Check sheet for the modelled part. Datum: model origin and axes. Units: mm. A direction names the side the tool comes from. Round coordinates to 2 decimals unless told otherwise and drop trailing zeros. Order: outer loops, then holes, each group sorted by start corner. A loop starts at its lowest first (then second) coordinate and runs counter-clockwise, first axis right, second up. Notation, with made-up numbers: (89.5, -2) -> (145.5, -2) arc R21 cw to (145.5, 8) -> close; hole circle Ø11 at (-5, 84). An arc over 180 degrees is marked (long way). Answer in a Markdown table with one row per item. Add a question column.
1. Draft check along Z on faces 4 (the flat face through (-1, 6, -22.23)), 5 (the flat face through (9.336, -0.986, 2.65)), 6 (the flat face through (38.655, 6, 0)), 7 (the cylindrical face through (26.151, 8.338, -18.804)). Enter one of: +Z half, -Z half, draft (parallel to the pull), parting line (faces both ways), or undercut.
2. Material ranges on L1, parallel to X at y = 9, z = -11 (3 decimals); L2, parallel to X at y = 6.25, z = -15.5 (3 decimals); L3, parallel to X at y = 13.75, z = -4.5 (3 decimals), recorded low to high. Write a range as from..to.
3. Sectioned sample at C-C, the plane z = 17. Record the boundary of the cut face in (x, y) (3 decimals), then the cut area to 3 significant figures.
4. Sectioned sample at D-D, the plane x = -14.5. Record the boundary of the cut face in (y, z).
5. Depth check by flat-ended pin: P1, Ø10, axis at x = 23.5, z = -15, coming from the -Y side; P2, Ø0.6, axis at x = 7, y = -1.5, coming from the +Z side; P3, Ø5, axis at x = -0.5, z = 16, coming from the +Y side. Enter the tip coordinate at first touch or a pass-through.
6. Sectioned sample at A-A, the plane z = -11. Record the boundary of the cut face in (x, y) (3 decimals).
7. Sectioned sample at B-B, the plane y = 3. Record the boundary of the cut face in (x, z) (3 decimals).
8. Access from +Z, -Z, +X, -X, +Y, -Y to the whole of each face (thin tool, end or side, straight path). Record for faces 1 (the flat face through (0, 8, 20.23)), 2 (the flat face through (30.655, 6, 0)), 3 (the flat face through (5.36, -0.99, 3.34)).
```python
from build123d import *

# Parameters (mm, degrees)
SKETCH1_W           = 59.31
SKETCH1_H           = 44.46
BOSS_EXTRUDE1_DEPTH = 2
SKETCH2_W           = 59.31
SKETCH2_H           = 44.46
SKETCH2_W_2         = 55.31
SKETCH2_H_2         = 40.46
BOSS_EXTRUDE2_DEPTH = 12.5
SKETCH3_W           = 1.5
SKETCH3_H           = 2.5
SKETCH5_W           = 6
SKETCH5_H           = 11.5
CUT_EXTRUDE1_DEPTH  = 10
BOSS_EXTRUDE3_DEPTH = 2
FILLET1_R           = 5
SKETCH7_W           = 10
SKETCH7_H           = 44.46
SKETCH7_W_2         = 6
SKETCH7_H_2         = 40.46
BOSS_EXTRUDE4_DEPTH = 12
FILLET2_R           = 3
FILLET3_R           = 0.25


with BuildPart() as part:
    # Sketch1 → Boss-Extrude1 (new body)
    with BuildSketch(Plane(origin=(0, 0, 0), x_dir=(1, 0, 0), z_dir=(0, 1, 0))):
        Rectangle(SKETCH1_W, SKETCH1_H)
    extrude(amount=BOSS_EXTRUDE1_DEPTH)

    # Sketch2 → Boss-Extrude2 (add)
    with BuildSketch(Plane(origin=(0, 2, 0), x_dir=(1, 0, 0), z_dir=(0, 1, 0))):
        Rectangle(SKETCH2_W, SKETCH2_H)
        Rectangle(SKETCH2_W_2, SKETCH2_H_2, mode=Mode.SUBTRACT)
    extrude(amount=BOSS_EXTRUDE2_DEPTH)

    # Cut-Sweep1: sweep along a path in Sketch4
    with BuildLine(Plane(origin=(0, 14.5, 0), x_dir=(1, 0, 0), z_dir=(0, 1, 0))) as cut_sweep1_path:
        Line((-29.655, -22.23), (29.655, -22.23))
        Line((29.655, -22.23), (29.655, 22.23))
        Line((29.655, 22.23), (-29.655, 22.23))
        Line((-29.655, 22.23), (-29.655, -22.23))
    # Sketch3 → Cut-Sweep1 (sweep, cut)
    with BuildSketch(Plane(origin=(29.655, 0, 0), x_dir=(0, 0, -1), z_dir=(1, 0, 0))):
        with Locations((-21.48, 13.25)):
            Rectangle(SKETCH3_W, SKETCH3_H)
    sweep(path=cut_sweep1_path.line, transition=Transition.RIGHT, mode=Mode.SUBTRACT)

    # Sketch5 → Cut-Extrude1 (cut)
    with BuildSketch(Plane(origin=(0, 0, 0), x_dir=(-1, 0, 0), z_dir=(0, -1, 0))):
        with Locations((21.655, 9.48)):
            Rectangle(SKETCH5_W, SKETCH5_H)
    extrude(amount=-CUT_EXTRUDE1_DEPTH, mode=Mode.SUBTRACT)

    # Sketch6 → Boss-Extrude3 (add)
    with BuildSketch(Plane.XZ):
        with BuildLine():
            Line((3.668359532, 11.043003806), (5.069466615, 11.043003806))
            Line((5.069466615, 11.043003806), (13.724692633, -5.981200546))
            add(Edge.make_bspline(
                [(13.724692633, -5.981200546), (13.770465415, -6.066255609), (13.860276332, -6.233142412), (14.049596398, -6.44471403), (14.259282132, -6.635498751), (14.514562764, -6.779774023), (14.797989941, -6.899882103), (15.118123905, -6.972877212), (15.467702486, -7.031048399), (15.713066528, -7.034166281), (15.841418927, -7.035797276)],
                knots=[0, 0, 0, 0, 0.923122777, 1.811262043, 2.707284477, 3.630407254, 4.607627564, 5.650245945, 6.770820012, 8, 8, 8, 8], degree=3))
            Line((15.841418927, -7.035797276), (16.587169471, -7.035797276))
            Line((16.587169471, -7.035797276), (16.587169471, -8))
            Line((16.587169471, -8), (6.704091546, -8))
            Line((6.704091546, -8), (6.704091546, -7.035797276))
            Line((6.704091546, -7.035797276), (7.491272677, -7.035797276))
            add(Edge.make_bspline(
                [(7.491272677, -7.035797276), (7.615561715, -7.034972065), (7.854152468, -7.033387954), (8.197254943, -7.024270941), (8.510837169, -6.998643255), (8.797935797, -6.976226749), (9.056099226, -6.935998597), (9.287242582, -6.897915489), (9.488634661, -6.845109649), (9.610791127, -6.800614432), (9.66826164, -6.779680927)],
                knots=[0, 0, 0, 0, 1.354335262, 2.59984206, 3.738199698, 4.78223889, 5.735982514, 6.583888141, 7.33376694, 8, 8, 8, 8], degree=3))
            add(Edge.make_bspline(
                [(9.66826164, -6.779680927), (9.734616654, -6.749406693), (9.857910933, -6.693154125), (9.99935023, -6.559441952), (10.092017823, -6.401790611), (10.10075551, -6.2849798), (10.105166, -6.226017644)],
                knots=[0, 0, 0, 0, 1.157571245, 2.15088362, 3.06662844, 4, 4, 4, 4], degree=3))
            add(Edge.make_bspline(
                [(10.105166, -6.226017644), (10.098921578, -6.149754311), (10.08575846, -5.988992716), (10.021947105, -5.840695302), (9.988407076, -5.762748366)],
                knots=[0, 0, 0, 0, 0.948775522, 2, 2, 2, 2], degree=3))
            Line((9.988407076, -5.762748366), (7.939476287, -1.732682292))
            Line((7.939476287, -1.732682292), (-1.495398027, -1.732682292))
            Line((-1.495398027, -1.732682292), (-2.666753681, -4.045262263))
            add(Edge.make_bspline(
                [(-2.666753681, -4.045262263), (-2.73463111, -4.18986222), (-2.860946743, -4.458953658), (-2.99975414, -4.849828516), (-3.097335174, -5.191789881), (-3.109447861, -5.40819885), (-3.114957291, -5.506632017)],
                knots=[0, 0, 0, 0, 1.244034282, 2.315069679, 3.233612959, 4, 4, 4, 4], degree=3))
            add(Edge.make_bspline(
                [(-3.114957291, -5.506632017), (-3.105178856, -5.610008506), (-3.085538794, -5.817640973), (-2.930679332, -6.11109022), (-2.683549261, -6.372065908), (-2.348052402, -6.608977598), (-1.921244388, -6.804306269), (-1.406472367, -6.937233956), (-0.80918362, -7.025851211), (-0.382171294, -7.032338986), (-0.154553614, -7.035797276)],
                knots=[0, 0, 0, 0, 0.676796425, 1.359350793, 2.130179084, 3.02304161, 4.041766613, 5.196580708, 6.505645488, 8, 8, 8, 8], degree=3))
            Line((-0.154553614, -7.035797276), (0.677824519, -7.035797276))
            Line((0.677824519, -7.035797276), (0.677824519, -8))
            Line((0.677824519, -8), (-8.241050681, -8))
            Line((-8.241050681, -8), (-8.241050681, -7.035797276))
            add(Edge.make_bspline(
                [(-8.241050681, -7.035797276), (-8.00595871, -7.030682959), (-7.560198321, -7.020985648), (-6.930404722, -6.931476506), (-6.376944833, -6.783238723), (-5.886269273, -6.568068877), (-5.442332689, -6.26093688), (-5.039212162, -5.844454164), (-4.645254972, -5.330344026), (-4.423041234, -4.933672593), (-4.305145029, -4.723217304)],
                knots=[0, 0, 0, 0, 1.157126977, 2.194040787, 3.123941644, 3.970721164, 4.81957436, 5.763811563, 6.813583119, 8, 8, 8, 8], degree=3))
            Line((-4.305145029, -4.723217304), (3.668359532, 11.043003806))
        make_face()
        Polygon((3.208856671, 7.570367432), (-1.009530248, -0.768479567), (7.446075674, -0.768479567), align=None, mode=Mode.SUBTRACT)
    extrude(amount=BOSS_EXTRUDE3_DEPTH)

    # Fillet1
    fillet1_edges = [part.edges().sort_by_distance(p)[0] for p in [
        (27.655, 8.25, 20.23),
        (27.655, 8.25, -20.23),
        (-27.655, 8.25, -20.23),
        (-27.655, 8.25, 20.23),
    ]]
    fillet(fillet1_edges, radius=FILLET1_R)

    # Sketch7 → Boss-Extrude4 (add)
    # profile 1 of 2: a face of its own
    with BuildSketch(Plane.XZ):
        with Locations((-33.655, 0)):
            Rectangle(SKETCH7_W, SKETCH7_H)
        with Locations((-33.655, 0)):
            Rectangle(SKETCH7_W_2, SKETCH7_H_2, mode=Mode.SUBTRACT)
    # profile 2 of 2: a face of its own
    with BuildSketch(Plane.XZ):
        with Locations((33.655, 0)):
            Rectangle(SKETCH7_W, SKETCH7_H)
        with Locations((33.655, 0)):
            Rectangle(SKETCH7_W_2, SKETCH7_H_2, mode=Mode.SUBTRACT)
    extrude(amount=-BOSS_EXTRUDE4_DEPTH)

    # Fillet2
    fillet2_edges = [part.edges().sort_by_distance(p)[0] for p in [
        (-28.155, 13.25, -20.73),
        (28.155, 13.25, -20.73),
        (28.155, 13.25, 20.73),
        (-28.155, 13.25, 20.73),
    ]]
    fillet(fillet2_edges, radius=FILLET2_R)

    # Fillet3
    fillet3_edges = [part.edges().sort_by_distance(p)[0] for p in [
        (-28.155, 12, 0),
        (0, 12, -20.73),
        (28.155, 12, 0),
        (0, 12, 20.73),
        (-27.276320344, 12, -19.851320344),
        (27.276320344, 12, -19.851320344),
        (27.276320344, 12, 19.851320344),
        (-27.276320344, 12, 19.851320344),
    ]]
    fillet(fillet3_edges, radius=FILLET3_R)


solid = part.part
```
Answer key:
| question | item | result |
|---|---|---|
| 1 | face 4 | -Z half |
| 1 | face 5 | +Z half |
| 1 | face 6 | draft |
| 1 | face 7 | undercut |
| 2 | L1 | x = -38.655..-36.655, -30.655..-27.655, 27.655..30.655, 36.655..38.655 |
| 2 | L2 | x = -38.655..-36.655, -30.655..-27.648, 27.648..30.655, 36.655..38.655 |
| 2 | L3 | x = -28.155..-27.655, 27.655..28.155 |
| 3 | outline | (-38.655, 0) -> (-36.655, 0) -> (-36.655, 12) -> (-38.655, 12) -> close; (-30.655, 0) -> (30.655, 0) -> (30.655, 12) -> (28.405, 12) arc R0.25 cw to (28.155, 12.25) -> (28.155, 14.5) -> (27.331, 14.5) -> (27.331, 2) -> (-27.331, 2) -> (-27.331, 14.5) -> (-28.155, 14.5) -> (-28.155, 12.25) arc R0.25 cw to (-28.405, 12) -> (-30.655, 12) -> close; (36.655, 0) -> (38.655, 0) -> (38.655, 12) -> (36.655, 12) -> close |
| 3 | area | 241 mm² |
| 4 | outline | (0, -22.23) -> (12, -22.23) -> (12, -20.98) arc R0.25 cw to (12.25, -20.73) -> (14.5, -20.73) -> (14.5, -20.23) -> (2, -20.23) -> (2, 20.23) -> (14.5, 20.23) -> (14.5, 20.73) -> (12.25, 20.73) arc R0.25 cw to (12, 20.98) -> (12, 22.23) -> (0, 22.23) -> close |
| 5 | P1 | stops at y = 0 |
| 5 | P2 | stops at z = 7.84 |
| 5 | P3 | stops at y = 2 |
| 6 | outline | (-38.655, 0) -> (-36.655, 0) -> (-36.655, 12) -> (-38.655, 12) -> close; (-30.655, 0) -> (-24.655, 0) -> (-24.655, 2) -> (-27.655, 2) -> (-27.655, 14.5) -> (-28.155, 14.5) -> (-28.155, 12.25) arc R0.25 cw to (-28.405, 12) -> (-30.655, 12) -> close; (-18.655, 0) -> (30.655, 0) -> (30.655, 12) -> (28.405, 12) arc R0.25 cw to (28.155, 12.25) -> (28.155, 14.5) -> (27.655, 14.5) -> (27.655, 2) -> (-18.655, 2) -> close; (36.655, 0) -> (38.655, 0) -> (38.655, 12) -> (36.655, 12) -> close |
| 7 | outline | (-38.655, -22.23) -> (38.655, -22.23) -> (38.655, 22.23) -> (-38.655, 22.23) -> close; hole (-36.655, -20.23) -> (-30.655, -20.23) -> (-30.655, 20.23) -> (-36.655, 20.23) -> close; hole (-27.655, -15.23) arc R5 ccw to (-22.655, -20.23) -> (22.655, -20.23) arc R5 ccw to (27.655, -15.23) -> (27.655, 15.23) arc R5 ccw to (22.655, 20.23) -> (-22.655, 20.23) arc R5 ccw to (-27.655, 15.23) -> close; hole (30.655, -20.23) -> (36.655, -20.23) -> (36.655, 20.23) -> (30.655, 20.23) -> close |
| 8 | face 1 | +Y |
| 8 | face 2 | +Y, -Y |
| 8 | face 3 | -Y |
